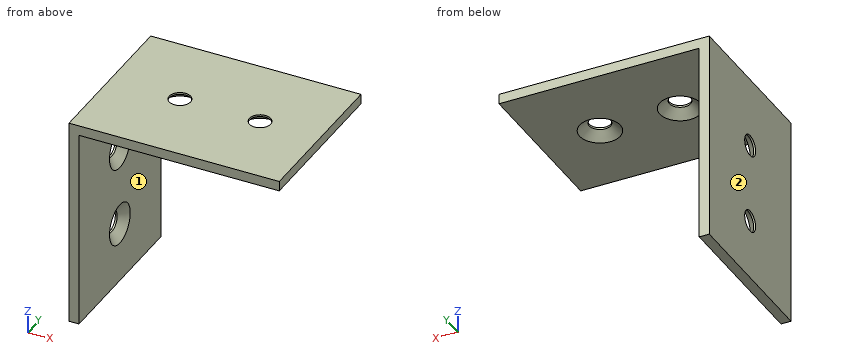
```python
from build123d import *

# Parameters (mm, degrees)
BOSS_EXTRUDE1_DEPTH                            = 50.8
CSK_FOR_1_4_FLAT_HEAD_MACHINE_SCREW_2_COUNT    = 2
CSK_FOR_1_4_FLAT_HEAD_MACHINE_SCREW_2_PITCH    = 25.4
CSK_FOR_1_4_FLAT_HEAD_MACHINE_SCREW_3_AT_COUNT = 2
CSK_FOR_1_4_FLAT_HEAD_MACHINE_SCREW_3_AT_PITCH = 25.4


with BuildPart() as part:
    # Sketch1 → Boss-Extrude1 (new body)
    with BuildSketch(Plane(origin=(0, 0, 0), x_dir=(1, 0, 0), z_dir=(0, 1, 0))):
        Polygon((0, 0), (0, 63.5), (3.175, 63.5), (3.175, 0), (66.675, 0), (66.675, -3.175), (0, -3.175), align=None)
    extrude(amount=BOSS_EXTRUDE1_DEPTH)

    # Sketch4 → CSK for 1_4 Flat Head Machine Screw _100 (revolve, cut)
    with BuildSketch(Plane(origin=(3.175, 25.4, -19.05), x_dir=(0, 0, -1), z_dir=(0, 1, 0))):
        Polygon((0, 0), (0, 3.175), (3.3782, 3.175), (3.3782, 2.568232241), (6.4389, 0), align=None)
    csk_for_1_4_flat_head_machine_screw_100 = revolve(axis=Axis((9.525, 25.4, -19.05), (-1, 0, 0)), mode=Mode.SUBTRACT)

    # CSK for 1_4 Flat Head Machine Screw  2: CSK for 1_4 Flat Head Machine Screw _100 ×2
    with Locations(*[(0, 0, -i * CSK_FOR_1_4_FLAT_HEAD_MACHINE_SCREW_2_PITCH) for i in range(1, CSK_FOR_1_4_FLAT_HEAD_MACHINE_SCREW_2_COUNT)]):
        add(csk_for_1_4_flat_head_machine_screw_100, mode=Mode.SUBTRACT)

    # Sketch6 → CSK for 1_4 Flat Head Machine Screw  3 (revolve, cut)
    with BuildSketch(Plane(origin=(47.625, 25.4, 0), x_dir=(0, 1, 0), z_dir=(1, 0, 0))):
        Polygon((0, 0), (0, 3.175), (3.3782, 3.175), (3.3782, 2.568232241), (6.4389, 0), align=None)
    csk_for_1_4_flat_head_machine_screw_3 = revolve(axis=Axis((47.625, 25.4, -6.35), (0, 0, 1)), mode=Mode.SUBTRACT)

    # CSK for 1_4 Flat Head Machine Screw 3 at: CSK for 1_4 Flat Head Machine Screw  3 ×2
    with Locations(*[(-i * CSK_FOR_1_4_FLAT_HEAD_MACHINE_SCREW_3_AT_PITCH, 0, 0) for i in range(1, CSK_FOR_1_4_FLAT_HEAD_MACHINE_SCREW_3_AT_COUNT)]):
        add(csk_for_1_4_flat_head_machine_screw_3, mode=Mode.SUBTRACT)


solid = part.part
```
The model under review builds one solid part; all positions refer to its coordinate system, in mm. Face numbers are marked on the shaded views. A direction names the side the tool comes from. Round coordinates to 2 decimals unless told otherwise and drop trailing zeros. Order: outer loops, then holes, each group sorted by start corner. A loop starts at its lowest first (then second) coordinate and runs counter-clockwise, first axis right, second up.
(1) Tool access review of the marked faces 1 and 2: name each direction out of +Z, -Z, +X, -X, +Y, -Y from which nothing blocks a thin tool from reaching the whole face with its end or side.
Working result:
face 1: -Z, +X, +Y, -Y
face 2: +Z, -Z, -X, +Y, -Y
(2) Take a section at D-D, the plane x = 32. State the section outline as (y, z) points (3 decimals).
Working result:
outline: (0, 0) - (50.8, 0) - (50.8, 3.175) - (0, 3.175) - close
(3) Wall thickness on L1, parallel to Z at x = 0.55, y = 25.4 (3 decimals); L2, parallel to Y at x = 0.4, z = -19.05; L3, parallel to Z at x = 17.5, y = 35 (3 decimals): over which ranges is each line inside the solid? List them lowest first.
Working result:
L1: z = -63.5 to -47.828, -41.072 to -22.428, -15.672 to 3.175
L2: y = 0 to 22.02, 28.78 to 50.8
L3: z = 0 to 3.175
(4) Take a section at B-B, the plane y = 25.4. Count the separate pieces of the cut face and the enclosed holes in it, plus the area to 3 significant figures.
Working result:
separate pieces: 5
enclosed holes: 0
area: 296 mm2
(5) Take a section at A-A, the plane z = -19.05. State the section outline as (x, y) points (3 decimals).
Working result:
outline: (0, 0) - (3.175, 0) - (3.175, 18.961) - (0.607, 22.022) - (0, 22.022) - close; (0, 28.778) - (0.607, 28.778) - (3.175, 31.839) - (3.175, 50.8) - (0, 50.8) - close
(6) For P1, Ø6, axis at y = 25.4, z = -19.05, coming from the +X side; P2, Ø15, axis at y = 30, z = -38, coming from the +X side (3 decimals); P3, Ø12, axis at x = 55.5, y = 33, coming from the -Z side, all flat-tipped, find the tip position at first contact; note any pin that passes through.
Working result:
P1: passes through
P2: stops at x = 3.175
P3: stops at z = 0
(7) Take a section at C-C, the plane y = 33. State the section outline as (x, z) points (3 decimals), plus the area to 3 significant figures.
Working result:
outline: (0, -63.5) - (3.175, -63.5) - (3.175, 0) - (66.675, 0) - (66.675, 3.175) - (0, 3.175) - close
area: 413 mm2
